Could you check a few things on this model? Use its own coordinates, in mm. A direction names the side the tool comes from. Give positions to 0.01 mm unless a question says otherwise; leave off trailing zeros. Write each loop counter-clockwise with the first axis right and the second up, starting at its lowest first coordinate (ties: lowest second). Pieces come first, ordered by that corner, then holes. Notation, with made-up numbers: M 14.25,8 L 33.25,8 A32 cw 33.25,46 Z; hole C 45.25,47 d3. An arc over 180 degrees is marked long. Use one line per item in the form item = value.
from build123d import *

# Parameters (mm, degrees)
BOSS_EXTRUDE1_DEPTH = 101.6
SKETCH6_R           = 12.7
CUT_EXTRUDE1_DEPTH  = 273.680564031
CUT_EXTRUDE5_DEPTH  = 285.565740427
SKETCH10_W          = 12.7
SKETCH10_H          = 12.7
CUT_EXTRUDE6_DEPTH  = 285.565740427
SKETCH11_W          = 25.4
SKETCH11_H          = 63.5
CUT_EXTRUDE7_DEPTH  = 206.591976072
CUT_EXTRUDE10_START = -25.4
SKETCH12_R          = 12.7
CUT_EXTRUDE10_DEPTH = 35.56


with BuildPart() as part:
    # Sketch5 → Boss-Extrude1 (new body)
    with BuildSketch(Plane(origin=(0, 130.175, 0), x_dir=(-1, 0, 0), z_dir=(0, 1, 0))):
        Polygon((-241.3, 0), (-190.5, 0), (-190.5, -25.4), (-101.6, -25.4), (-101.6, -76.2), (-228.6, -76.2), (-228.6, -63.5), (-241.3, -63.5), align=None)
    extrude(amount=-BOSS_EXTRUDE1_DEPTH)

    # Sketch6 → Cut-Extrude1 (cut, through all)
    with BuildSketch(Plane(origin=(0, 130.175, 0), x_dir=(-1, 0, 0), z_dir=(0, 1, 0))):
        with Locations(Location((-139.7, -50.8, 0), (0, 0, 90))):
            Circle(SKETCH6_R)
    extrude(amount=-CUT_EXTRUDE1_DEPTH, mode=Mode.SUBTRACT)

    # Sketch8 → Cut-Extrude5 (cut, through all)
    with BuildSketch(Plane.XY):
        Polygon((190.5, 104.775), (139.7, 104.775), (127, 104.775), (101.6, 104.775), (101.6, 28.575), (190.5, 28.575), (190.5, 92.075), align=None)
    extrude(amount=-CUT_EXTRUDE5_DEPTH, mode=Mode.SUBTRACT)

    # Sketch10 → Cut-Extrude6 (cut, through all)
    with BuildSketch(Plane.XY):
        with Locations((234.95, 123.825)):
            Rectangle(SKETCH10_W, SKETCH10_H)
    extrude(amount=-CUT_EXTRUDE6_DEPTH, mode=Mode.SUBTRACT)

    # Sketch11 → Cut-Extrude7 (cut, through all)
    with BuildSketch(Plane(origin=(241.3, 0, 0), x_dir=(0, 0, -1), z_dir=(1, 0, 0))):
        with Locations((12.7, 60.325)):
            Rectangle(SKETCH11_W, SKETCH11_H)
    extrude(amount=-CUT_EXTRUDE7_DEPTH, mode=Mode.SUBTRACT)

    # Sketch12 → Cut-Extrude10 (cut)
    with BuildSketch(Plane.XY.offset(CUT_EXTRUDE10_START)):
        with Locations((215.9, 53.975)):
            Circle(SKETCH12_R)
    extrude(amount=-CUT_EXTRUDE10_DEPTH, mode=Mode.SUBTRACT)


solid = part.part
1) Thinking about a two-plate mould opening in X: for faces 1 (the flat face through (216, 92.075, -13)), 2 (the cylindrical face through (152.292, 117.653, -52.453)), 3 (the flat face through (101.6, 118, -50)), which applies, released by +X, released by -X, zero draft, split by the parting line, or undercut?
Checked values:
face_1 = zero draft
face_2 = undercut
face_3 = released by -X
2) I want a section at D-D, the plane x = 215.9. Please give me the cut outline in (y, z) (3 decimals), plus the area to 3 significant figures.
Checked values:
outline = M 28.575,-76.2 L 130.175,-76.2 L 130.175,0 L 92.075,0 L 92.075,-25.4 L 66.675,-25.4 L 66.675,-60.96 L 41.275,-60.96 L 41.275,-25.4 L 28.575,-25.4 Z
area = 5,230 mm2
3) For faces 4 (the cylindrical face through (206.54, 62.56, -42.93)), 5 (the flat face through (147, 118, -25.4)), 6 (the flat face through (235, 117.475, -31)), 7 (the flat face through (235, 74, -63.5)), 8 (the flat face through (157, 104.775, -50)), which set-ups out of +Z, -Z, +X, -X, +Y, -Y let a thin tool reach every point of the face, with its end or its side?
Checked values:
face_4 = +Z
face_5 = +Z, -X, +Y, -Y
face_6 = +Z, -Z, +X, +Y
face_7 = -Z, +X, +Y, -Y
face_8 = +Z, -Z, -X, -Y
4) I want a section at B-B, the plane x = 139.7. Please give me the cut outline in (y, z) (3 decimals).
Checked values:
outline = M 104.775,-76.2 L 130.175,-76.2 L 130.175,-63.5 L 104.775,-63.5 Z; M 104.775,-38.1 L 130.175,-38.1 L 130.175,-25.4 L 104.775,-25.4 Z
5) I want a section at C-C, the plane y = 84. Please give me the cut outline in (x, z).
Checked values:
outline = M 190.5,-76.2 L 228.6,-76.2 L 228.6,-63.5 L 241.3,-63.5 L 241.3,-25.4 L 190.5,-25.4 Z
6) For pin 1 Ø6.5 at (x, z) = (235.5, -29.5) entering from +Y (3 decimals); pin 2 Ø5 at (x, y) = (213, 62) entering from +Z; pin 3 Ø7.5 at (x, z) = (227, -16) entering from -Y (3 decimals), each with a flat end and sliding along its axis, tell me the tip position at first contact or that it passes through.
Checked values:
pin_1 = 117.475
pin_2 = -60.96
pin_3 = 92.075
7) If I drill on L1, parallel to Z at x = 139, y = 124; L2, parallel to Y at x = 215, z = -37 (3 decimals); L3, parallel to X at y = 122, z = -50.8, over which ranges is the centre line in solid material (lowest first)?
Checked values:
L1 = -76.2 to -63.48, -38.12 to -25.4
L2 = 28.575 to 41.307, 66.643 to 130.175
L3 = 101.6 to 127, 152.4 to 228.6
8) I want a section at A-A, the plane z = -50.8. Please give me the cut outline in (x, y) (3 decimals), plus the area to 3 significant figures.
Checked values:
outline = M 101.6,104.775 L 127,104.775 L 127,130.175 L 101.6,130.175 Z; M 152.4,104.775 L 190.5,104.775 L 190.5,28.575 L 241.3,28.575 L 241.3,117.475 L 228.6,117.475 L 228.6,130.175 L 152.4,130.175 Z; hole C 215.9,53.975 d25.4
area = 6,110 mm2
